Verification items for the finished model (mm, model axes). A direction names the side the tool comes from. Give positions to 0.01 mm unless a question says otherwise; leave off trailing zeros. Loops run counter-clockwise (first coordinate to the right, second up) from the corner with the lowest first, then second, coordinate; pieces in that order, holes last. Notation, with made-up numbers: (20.25, 51.25) - (44.25, 51.25) arc R23 cw to (44.25, 70.25) - close; hole circle Ø2 at (70.25, 46). An arc over 180 degrees is marked (long way). One line per item, written item: value. Start each with the question number.
1. Sectioned sample at C-C (z = -75). Record the cut outline in (x, y).
2. Sectioned sample at D-D (x = 0). Record the cut outline in (y, z), plus the area to 3 significant figures.
3. Mould release check, pull along Y, two halves, no side actions. Record for faces 1 (the flat face through (-137, 0, 114.7)), 2 (the flat face through (-1, -31.75, -117)), 3 (the cylindrical face through (144.37, -13.97, 117.92)), 4 (the cylindrical face through (-132.256, -13.968, 117.919)): pulls with the +Y half, pulls with the -Y half, needs draft (parallel to the pull), parting line crosses it, or undercut.
4. Sectioned sample at B-B (y = -0.5). Record the cut outline in (x, z).
5. Scan lines: L1, parallel to X at y = -28, z = -1.5; L2, parallel to X at y = -6.5, z = -47.5; L3, parallel to Z at x = -127, y = 14.5. Record each from-to range of solid material in increasing order. Write a range as [from, to].
6. Sectioned sample at A-A (z = 44). Record the cut outline in (x, y), plus the area to 3 significant figures.
7. Gauge pin test, flat ends, axial feed: pin 1 (7.5 mm diameter, centred on x = 138.31, y = 15.88, fed in from +Z); pin 2 (5 mm diameter, centred on x = -69.5, y = -1, fed in from +Z); pin 3 (9.5 mm diameter, centred on x = 141, y = 12, fed in from -Z); pin 4 (8 mm diameter, centred on y = 0.5, z = 59.5, fed in from +X). Record the tip position at first contact, or that the pin passes through.
8. Access from +Z, -Z, +X, -X, +Y, -Y to the whole of each face (thin tool, end or side, straight path). Record for faces 5 (the flat face through (137, 0, 114.7)), 6 (the flat face through (114.7, 0, 60)), 7 (the flat face through (-121.05, 0, 57)).
from build123d import *

# Parameters (mm, degrees)
BOSS_EXTRUDE1_DEPTH = 31.75
SKETCH15_R          = 6.35
CUT_EXTRUDE1_DEPTH  = 288.83021471


with BuildPart() as part:
    # Sketch1 → Boss-Extrude1 (new, symmetric)
    with BuildSketch(Plane(origin=(0, 0, 0), x_dir=(1, 0, 0), z_dir=(0, 1, 0))):
        with BuildLine():
            Line((-114.7, -121.05), (-114.7, 0))
            ThreePointArc((-114.7, 0), (0, 114.7), (114.7, 0))
            Line((114.7, 0), (114.7, -121.05))
            Line((114.7, -121.05), (152.4, -121.05))
            Line((152.4, -121.05), (152.4, -114.7))
            Line((152.4, -114.7), (121.05, -114.7))
            Line((121.05, -114.7), (121.05, 0))
            ThreePointArc((121.05, 0), (0, 121.05), (-121.05, 0))
            Line((-121.05, 0), (-121.05, -12.7))
            Line((-121.05, -12.7), (-121.05, -114.7))
            Line((-121.05, -114.7), (-152.4, -114.7))
            Line((-152.4, -114.7), (-152.4, -121.05))
            Line((-152.4, -121.05), (-114.7, -121.05))
        make_face()
    extrude(amount=BOSS_EXTRUDE1_DEPTH, both=True)

    # Sketch15 → Cut-Extrude1 (cut, through all)
    with BuildSketch(Plane.XY.offset(121.05)):
        with Locations((-138.3125, 15.875)):
            Circle(SKETCH15_R)
        with Locations((-138.3125, -15.875)):
            Circle(SKETCH15_R)
        with Locations((138.3125, -15.875)):
            Circle(SKETCH15_R)
        with Locations((138.3125, 15.875)):
            Circle(SKETCH15_R)
    extrude(amount=-CUT_EXTRUDE1_DEPTH, mode=Mode.SUBTRACT)


solid = part.part
Results are:
1. outline: (-95.02, -31.75) - (-86.78, -31.75) - (-86.78, 31.75) - (-95.02, 31.75) - close; (86.78, -31.75) - (95.02, -31.75) - (95.02, 31.75) - (86.78, 31.75) - close
2. outline: (-31.75, -121.05) - (31.75, -121.05) - (31.75, -114.7) - (-31.75, -114.7) - close
2. area: 403 mm^2
3. face 1: needs draft
3. face 2: pulls with the -Y half
3. face 3: undercut
3. face 4: undercut
4. outline: (-152.4, 114.7) - (-121.05, 114.7) - (-121.05, 0) arc R121.05 ccw to (121.05, 0) - (121.05, 114.7) - (152.4, 114.7) - (152.4, 121.05) - (114.7, 121.05) - (114.7, 0) arc R114.7 cw to (-114.7, 0) - (-114.7, 121.05) - (-152.4, 121.05) - close
5. L1: x = [-121.04, -114.69], [114.69, 121.04]
5. L2: x = [-111.34, -104.4], [104.4, 111.34]
5. L3: z = [114.7, 121.05]
6. outline: (-121.05, -31.75) - (-114.7, -31.75) - (-114.7, 31.75) - (-121.05, 31.75) - close; (114.7, -31.75) - (121.05, -31.75) - (121.05, 31.75) - (114.7, 31.75) - close
6. area: 806 mm^2
7. pin 1: passes through
7. pin 2: stops at z = -89.29
7. pin 3: stops at z = 114.7
7. pin 4: stops at x = 121.05
8. face 5: -Z, +X, +Y, -Y
8. face 6: +Z, +Y, -Y
8. face 7: -Z, -X, +Y, -Y
